from build123d import *

# Parameters (mm, degrees)
ESQUISSE1_R        = 5
BOSS_EXTRU_1_DEPTH = 35
ESQUISSE3_R        = 10
BOSS_EXTRU_2_DEPTH = 3
CONG_1_R           = 0.5


with BuildPart() as part:
    # Esquisse1 → Boss.-Extru.1 (new body)
    with BuildSketch(Plane.XY):
        Circle(ESQUISSE1_R)
    extrude(amount=BOSS_EXTRU_1_DEPTH)

    # Esquisse3 → Boss.-Extru.2 (add)
    with BuildSketch(Plane.XY.offset(35)):
        Circle(ESQUISSE3_R)
    extrude(amount=BOSS_EXTRU_2_DEPTH)

    # Congé1
    cong_1_edges = [part.edges().sort_by_distance(p)[0] for p in [
        (-5, 0, 35),
    ]]
    fillet(cong_1_edges, radius=CONG_1_R)


solid = part.part
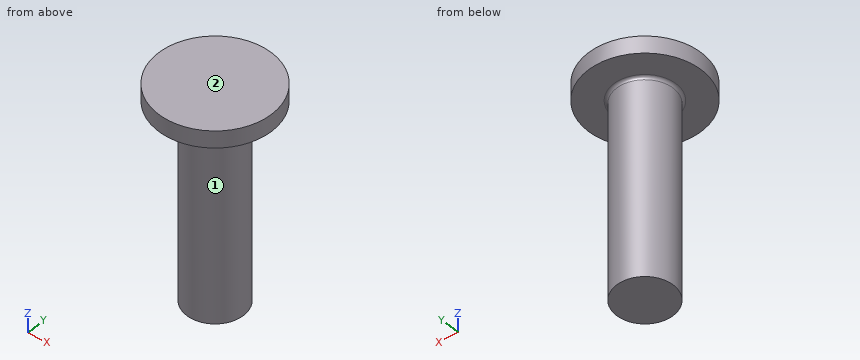
The listing builds one solid part. Answer for the finished solid, in the listing's coordinates (mm). Face numbers are marked on the shaded views. A direction names the side the tool comes from. Round coordinates to 2 decimals unless told otherwise and drop trailing zeros. Order: outer loops, then holes, each group sorted by start corner. A loop starts at its lowest first (then second) coordinate and runs counter-clockwise, first axis right, second up. Notation, with made-up numbers: (-28, -26) -> (-19, -26) arc R23 ccw to (-19, 8) -> close; hole circle Ø7 at (29, 60.5). An arc over 180 degrees is marked (long way). One line per item, written item: value.
Item 1: Straight lines are drawn through the part: L1, parallel to Z at x = -8.25, y = -2.5; L2, parallel to Y at x = 1, z = 33; L3, parallel to X at y = 2.5, z = 31.5. For each, find the intervals that lie inside material, in ascending order.
Taken from the geometry:
L1: z = 35 to 38
L2: y = -4.9 to 4.9
L3: x = -4.33 to 4.33
Item 2: For the marked faces 1 and 2, determine the directions among +Z, -Z, +X, -X, +Y, -Y from which every point of the face is accessible in a straight line to the end or side of a thin tool.
Taken from the geometry:
face 1: -Z
face 2: +Z, +X, -X, +Y, -Y
Item 3: Find section D-D, the plane y = -6.25. Give the vertices of the cut face in (x, z), then the cut area to 3 significant figures.
Taken from the geometry:
outline: (-7.81, 35) -> (7.81, 35) -> (7.81, 38) -> (-7.81, 38) -> close
area: 46.8 mm2
Item 4: Given P1, Ø10, axis at y = -8, z = 14.5, coming from the +X side; P2, Ø3, axis at x = -3, z = 14, coming from the -Y side; P3, Ø4, axis at x = 1, z = 21.5, coming from the -Y side; P4, Ø2, axis at x = -6.5, z = 11, coming from the -Y side, each flat-ended and moving along its own axis, determine where each tip first touches the part or whether it passes through.
Taken from the geometry:
P1: stops at x = 4
P2: stops at y = -4.77
P3: stops at y = -5
P4: passes through
Item 5: Find section A-A, the plane x = 0. Give the vertices of the cut face in (y, z), then the cut area to 3 significant figures.
Taken from the geometry:
outline: (-10, 35) -> (-5.5, 35) arc R0.5 cw to (-5, 34.5) -> (-5, 0) -> (5, 0) -> (5, 34.5) arc R0.5 cw to (5.5, 35) -> (10, 35) -> (10, 38) -> (-10, 38) -> close
area: 410 mm2
Item 6: Find section C-C, the plane z = 6.5. Give the vertices of the cut face in (x, y), then the cut area to 3 significant figures.
Taken from the geometry:
outline: circle Ø10 at (0, 0)
area: 78.5 mm2
